from build123d import *

# Parameters (mm, degrees)
EXTRUDE1_DEPTH = 200
SKETCH2_W      = 110
SKETCH2_H      = 80
EXTRUDE2_DEPTH = 200
SKETCH3_W      = 50
SKETCH3_H      = 60
EXTRUDE3_DEPTH = 180
SKETCH4_R      = 260
EXTRUDE4_DEPTH = 0.01


with BuildPart() as part:
    # Sketch1 → Extrude1 (new body)
    with BuildSketch(Plane.XY):
        Polygon((-60, 200), (0, 100), (110, 70), (110, 0), (0, 0), (-120, 0), (-120, 100), align=None)
    extrude(amount=EXTRUDE1_DEPTH)

    # Sketch2 → Extrude2 (cut)
    with BuildSketch(Plane(origin=(0, 0, 0), x_dir=(1, 0, 0), z_dir=(0, 1, 0))):
        with Locations((55, -160)):
            Rectangle(SKETCH2_W, SKETCH2_H)
    extrude(amount=EXTRUDE2_DEPTH, mode=Mode.SUBTRACT)

    # Sketch3 → Extrude3 (add)
    with BuildSketch(Plane(origin=(0, 0, 0), x_dir=(1, 0, 0), z_dir=(0, 1, 0))):
        with Locations((-145, -30)):
            Rectangle(SKETCH3_W, SKETCH3_H)
    extrude(amount=EXTRUDE3_DEPTH)

    # Sketch4 → Extrude4 (add)
    with BuildSketch(Plane(origin=(0, 0, 0), x_dir=(1, 0, 0), z_dir=(0, 1, 0))):
        with Locations(Location((-30, -99.759965953, 0), (0, 0, 270))):  # turned: the seam where the file's is
            Circle(SKETCH4_R)
    extrude(amount=EXTRUDE4_DEPTH)


solid = part.part
Geometry check sheet. Reference: the model listing, model coordinates, mm. A direction names the side the tool comes from. Give positions to 0.01 mm unless a question says otherwise; leave off trailing zeros. Write each loop counter-clockwise with the first axis right and the second up, starting at its lowest first coordinate (ties: lowest second). Pieces come first, ordered by that corner, then holes.
1) Cross-section at A-A (y = 145). Record the boundary of the cut face in (x, z).
Values follow:
outline: (-170, 0) - (-120, 0) - (-120, 60) - (-170, 60) - close; (-93, 0) - (-27, 0) - (-27, 200) - (-93, 200) - close
2) Go/stop test with flat-tipped pins: pin 1 Ø25 at (x, y) = (-133.5, 83) entering from +Z; pin 2 Ø15 at (x, z) = (-144, 21) entering from +Y; pin 3 Ø8 at (y, z) = (51, 78.5) entering from -X. Record where each tip stops, or that it passes through.
Values follow:
pin 1: stops at z = 60
pin 2: stops at y = 180
pin 3: stops at x = -120
3) Cross-section at C-C (y = 110.5). Record the boundary of the cut face in (x, z), plus the area to 3 significant figures.
Values follow:
outline: (-170, 0) - (-120, 0) - (-120, 60) - (-170, 60) - close; (-113.7, 0) - (-6.3, 0) - (-6.3, 200) - (-113.7, 200) - close
area: 24,500 mm2
4) Thickness scan on line 1 (Z direction, x = -74.5, y = 41); line 2 (Z direction, x = 13.5, y = 52); line 3 (X direction, y = 16.5, z = 137). Record the ranges inside material, lowest first.
Values follow:
line 1: z = 0 to 200
line 2: z = 0 to 120
line 3: x = -120 to 0
5) Set-up check for faces 1 (the face through (54, 38, 120)), 2 (the face through (-145, 180, 30)), 3 (the face through (110, 35, 59)), 4 (the face through (-59, 79, 200)), 5 (the face through (-145, 89, 60)): record each of +Z, -Z, +X, -X, +Y, -Y from which the full face is reachable in a straight line by a thin tool's end or side.
Values follow:
face 1: +Z, +X, +Y
face 2: +Z, -Z, -X, +Y
face 3: +Z, -Z, +X, +Y
face 4: +Z, +X, -X, +Y
face 5: +Z, -X, +Y
6) Release check for a two-part mould opening along X. For faces 6 (the face through (-63, 76, 0)), 7 (the face through (-120, 139, 30)), 8 (the face through (-170, 89, 30)), 9 (the face through (-30.42, 150.7, 98.6)) record: released by +X, released by -X, zero draft, split by the parting line, or undercut.
Values follow:
face 6: zero draft
face 7: undercut
face 8: released by -X
face 9: released by +X
